The figure shows three views and two pictorial views of one solid part (mm, origin at its lowest corner). Answer the questions. A direction names the side the tool comes from. Coordinates: 2 decimals unless noted, no trailing zeros. Loops run counter-clockwise (first coordinate to the right, second up) from the corner with the lowest first, then second, coordinate; pieces in that order, holes last. Notation, with made-up numbers: M 2.5,-1 L 46.5,-1 A3 ccw 46.5,4 Z; hole C 68.5,33.25 d10. An arc over 180 degrees is marked long. One line per item, written item: value. Start each with the question number.
1. Determine the mould class of the marked faces 3, 4 and 5 for opening direction Y: +Y half, -Y half, draft (parallel to the pull), parting line (faces both ways), or undercut.
2. The part is cut by section D-D (x = 0.9). Write down the section's boundary in (y, z).
3. For the marked faces 1 and 2, determine the directions among +Z, -Z, +X, -X, +Y, -Y from which every point of the face is accessible in a straight line to the end or side of a thin tool.
4. Consider probe 1 along Z at (x, y) = (1.8, 3.95); probe 2 along Z at (x, y) = (3.1, 3.2); probe 3 along Y at (x, z) = (3.3, 8) (1 decimal). Determine where each line is inside the solid, lowest interval first.
5. The part is cut by section C-C (y = 3.7). Write down the section's boundary in (x, z).
6. Flat-ended cylindrical pins translate along their axes: pin 1 (1.5 mm diameter, centred on y = 4.5, z = 7, fed in from -X); pin 2 (1 mm diameter, centred on y = 0.5, z = 15, fed in from -X) (1 decimal). Find the tip coordinate at first contact, or state that the pin passes through.
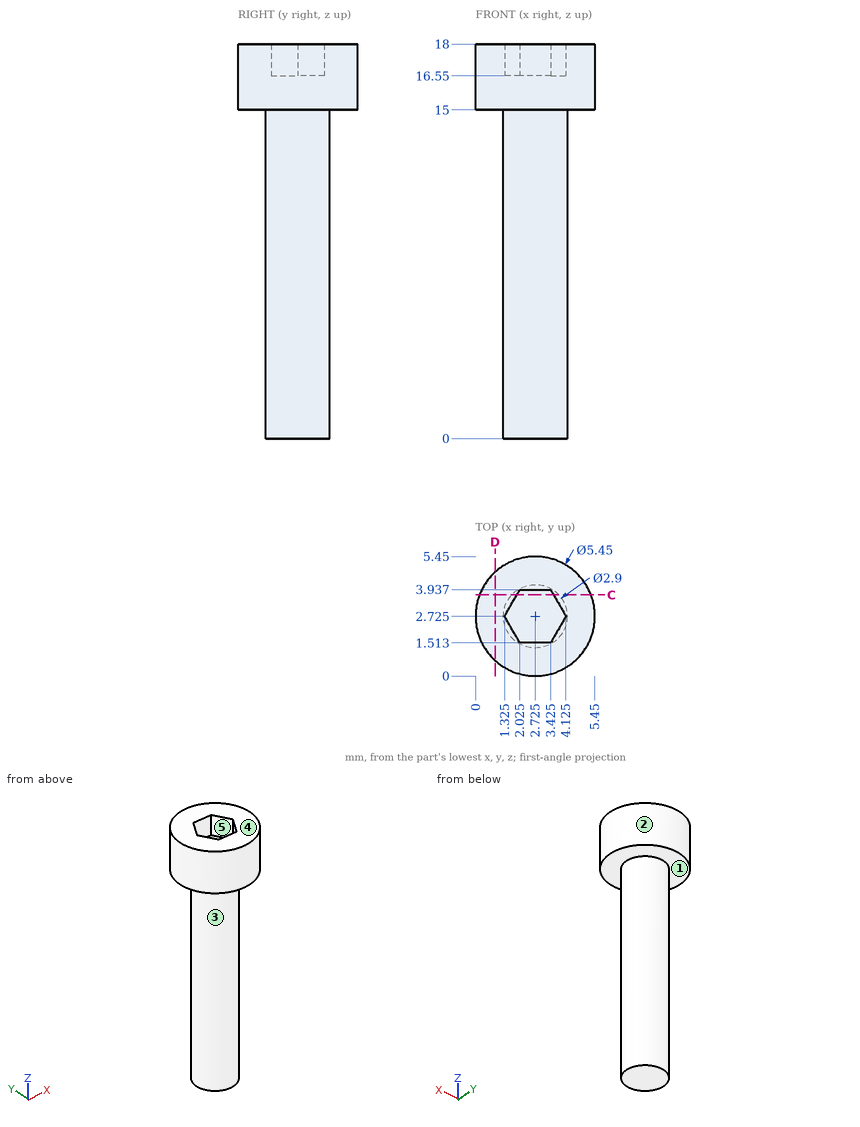
Answer block:
1. face 3: parting line
1. face 4: draft
1. face 5: undercut
2. outline: M 0.7,15 L 4.75,15 L 4.75,18 L 0.7,18 Z
3. face 1: -Z
3. face 2: +Z, -Z
4. probe 1: z = 15 to 18
4. probe 2: z = 0 to 16.55
4. probe 3: y = 1.4 to 4.1
5. outline: M 0.18,15 L 1.65,15 L 1.65,0 L 3.8,0 L 3.8,15 L 5.27,15 L 5.27,18 L 3.56,18 L 3.56,16.55 L 1.89,16.55 L 1.89,18 L 0.18,18 Z
6. pin 1: stops at x = 1.7
6. pin 2: stops at x = 0.6
